```python
from build123d import *

# Parameters (mm, degrees)
F0_W      = 70
F0_H      = 70
F1_DEPTH  = 120
F3_D      = 13.49248
F4_D      = 8.8
F4_DEPTH  = 20
F4_TIP    = 2.6437867237
F2_R      = 15.05
F5_DEPTH  = 1.2
F7_D      = 8.8
F7_DEPTH  = 20
F7_TIP    = 2.6437867237
F6_R      = 15.05
F8_DEPTH  = 1.2
F10_D     = 5.5
F10_DEPTH = 20
F10_TIP   = 1.6523667023
F12_D     = 8.8
F12_DEPTH = 20
F12_TIP   = 2.6437867237
F14_D     = 10.0838
F14_DEPTH = 40
F14_TIP   = 3.0294791551
F13_R     = 13.75
F15_DEPTH = 1.2
F16_R     = 15.5
F17_DEPTH = 2


with BuildPart() as f1:
    # F0 (on Right) → F1 (new body)
    with BuildSketch(Plane.YZ):
        Rectangle(F0_W, F0_H)
    extrude(amount=F1_DEPTH)

    # F3 (through all)
    with Locations(Plane.YZ.offset(120)):
        with Locations((-19, 0), (19, 0)):
            Hole(F3_D / 2)

    # F4
    with Locations(Plane.YZ.offset(120)):
        with Locations((-26, 26), (26, 25.9378720075), (-18, -26), (18, -26)):
            Hole(F4_D / 2, depth=F4_DEPTH)
            with Locations((0, 0, -(F4_DEPTH + F4_TIP / 2))):  # 118° drill point
                Cone(0, F4_D / 2, F4_TIP, mode=Mode.SUBTRACT)

    # F2 (on face) → F5 (cut)
    with BuildSketch(Plane.YZ.offset(120)):
        with Locations((-19, 0)):
            Circle(F2_R)
        with Locations((19, 0)):
            Circle(F2_R)
    extrude(amount=-F5_DEPTH, mode=Mode.SUBTRACT)

    # F7
    with Locations(Plane(origin=(0, 0, 0), x_dir=(0, -1, 0), z_dir=(-1, 0, 0))):
        with Locations((-26, 25.9378720075), (26, 26), (-18, -26), (18, -26)):
            Hole(F7_D / 2, depth=F7_DEPTH)
            with Locations((0, 0, -(F7_DEPTH + F7_TIP / 2))):  # 118° drill point
                Cone(0, F7_D / 2, F7_TIP, mode=Mode.SUBTRACT)

    # F6 (on face) → F8 (cut)
    with BuildSketch(Plane(origin=(0, 0, 0), x_dir=(0, -1, 0), z_dir=(-1, 0, 0))):
        with Locations((-19, 0)):
            Circle(F6_R)
        with Locations((19, 0)):
            Circle(F6_R)
    extrude(amount=-F8_DEPTH, mode=Mode.SUBTRACT)

    # F10
    with Locations(Plane.XY.offset(35)):
        with Locations((19.5, 20.25), (19.5, -20.25), (50.5, -20.25), (50.5, 20.25), (69.5, 20.25), (69.5, -20.25), (100.5, -20.25), (100.5, 20.25)):
            Hole(F10_D / 2, depth=F10_DEPTH)
            with Locations((0, 0, -(F10_DEPTH + F10_TIP / 2))):  # 118° drill point
                Cone(0, F10_D / 2, F10_TIP, mode=Mode.SUBTRACT)

    # F12
    with Locations(Plane(origin=(0, 0, -35), x_dir=(1, 0, 0), z_dir=(0, 0, -1))):
        with Locations((8, 27), (8, -27), (112, 27), (112, -27)):
            Hole(F12_D / 2, depth=F12_DEPTH)
            with Locations((0, 0, -(F12_DEPTH + F12_TIP / 2))):  # 118° drill point
                Cone(0, F12_D / 2, F12_TIP, mode=Mode.SUBTRACT)

    # F14
    with Locations(Plane(origin=(0, 35, 0), x_dir=(-1, 0, 0), z_dir=(0, 1, 0))):
        with Locations((-85, 19), (-35, 19), (-35, -19), (-85, -19)):
            Hole(F14_D / 2, depth=F14_DEPTH)
            with Locations((0, 0, -(F14_DEPTH + F14_TIP / 2))):  # 118° drill point
                Cone(0, F14_D / 2, F14_TIP, mode=Mode.SUBTRACT)

    # F13 (on face) → F15 (cut)
    with BuildSketch(Plane(origin=(0, 35, 0), x_dir=(-1, 0, 0), z_dir=(0, 1, 0))):
        with Locations((-85, 19)):
            Circle(F13_R)
        with Locations((-85, -19)):
            Circle(F13_R)
        with Locations((-35, 19)):
            Circle(F13_R)
        with Locations((-35, -19)):
            Circle(F13_R)
    extrude(amount=-F15_DEPTH, mode=Mode.SUBTRACT)

    # F16 (on face) → F17 (cut)
    with BuildSketch(Plane.XZ.offset(35)):
        with Locations((67.5, -19)):
            Circle(F16_R)
    extrude(amount=-F17_DEPTH, mode=Mode.SUBTRACT)


solid = f1.part
```
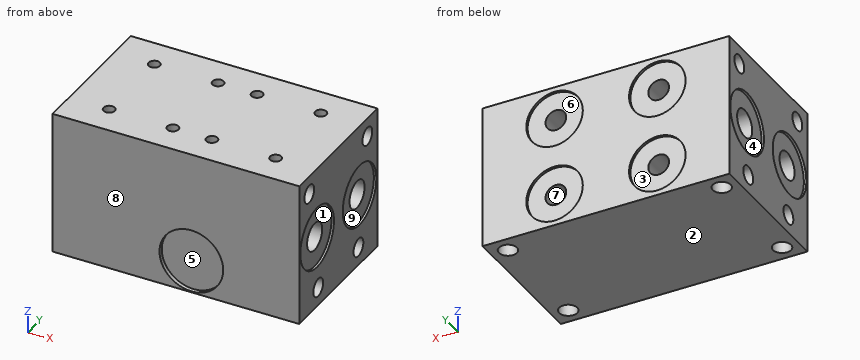
Verification items for the finished model (mm, model axes). Face numbers are marked on the shaded views. A direction names the side the tool comes from. Give positions to 0.01 mm unless a question says otherwise; leave off trailing zeros. Order: outer loops, then holes, each group sorted by start corner. A loop starts at its lowest first (then second) coordinate and runs counter-clockwise, first axis right, second up. Notation, with made-up numbers: (47, -23.75) -> (82, -23.75) arc R17 ccw to (82, -14.75) -> close; hole circle Ø6 at (68.25, 6). An arc over 180 degrees is marked (long way). One line per item, written item: value.
(1) Scan lines: line 1 along X through (y, z) = (-20, 28); line 2 along Y through (x, z) = (14, 29); line 3 along Y through (x, z) = (21, -27.5). Record each from-to range of solid material in increasing order. Write a range as [from, to].
Final values:
line 1: [0, 16.76], [22.24, 47.76], [53.24, 66.76], [72.24, 97.76], [103.24, 120]
line 2: [-35, -29.22], [-22.78, 22.84], [29.16, 35]
line 3: [-35, -20.29], [-15.71, 15.71], [20.29, 35]
(2) Sectioned sample at B-B on x = 24. Record the cut outline in (y, z), then the cut area to 3 significant figures.
Final values:
outline: (-35, -35) -> (35, -35) -> (35, -27.25) -> (33.8, -27.25) -> (33.8, -10.75) -> (35, -10.75) -> (35, 10.75) -> (33.8, 10.75) -> (33.8, 27.25) -> (35, 27.25) -> (35, 35) -> (-35, 35) -> close; hole circle Ø13.49 at (-19, 0); hole circle Ø13.49 at (19, 0)
area: 4,570 mm^2
(3) Sectioned sample at C-C on y = 28.5. Count the separate pieces of the cut face and the enclosed holes in it, then the cut area to 3 significant figures.
Final values:
separate pieces: 1
enclosed holes: 4
area: 7,380 mm^2
(4) Sectioned sample at A-A on z = 0. Record the cut outline in (x, y), then the cut area to 3 significant figures.
Final values:
outline: (0, -35) -> (120, -35) -> (120, -34.05) -> (118.8, -34.05) -> (118.8, -25.75) -> (1.2, -25.75) -> (1.2, -34.05) -> (0, -34.05) -> close; (0, -3.95) -> (1.2, -3.95) -> (1.2, -12.25) -> (118.8, -12.25) -> (118.8, -3.95) -> (120, -3.95) -> (120, 3.95) -> (118.8, 3.95) -> (118.8, 12.25) -> (1.2, 12.25) -> (1.2, 3.95) -> (0, 3.95) -> close; (0, 34.05) -> (1.2, 34.05) -> (1.2, 25.75) -> (118.8, 25.75) -> (118.8, 34.05) -> (120, 34.05) -> (120, 35) -> (0, 35) -> close
area: 5,080 mm^2
(5) Gauge pin test, flat ends, axial feed: pin 1 (7 mm diameter, centred on y = -26, z = 26, fed in from -X); pin 2 (24 mm diameter, centred on y = 19, z = 0, fed in from -X); pin 3 (22 mm diameter, centred on x = 35, z = -19, fed in from +Y). Record the tip position at first contact, or that the pin passes through.
Final values:
pin 1: x = 20.54
pin 2: x = 1.2
pin 3: y = 33.8
(6) Sectioned sample at D-D on x = 41.5. Record the cut outline in (y, z), then the cut area to 3 significant figures.
Final values:
outline: (-35, -35) -> (35, -35) -> (35, -31.12) -> (33.8, -31.12) -> (33.8, -6.88) -> (35, -6.88) -> (35, 6.88) -> (33.8, 6.88) -> (33.8, 31.12) -> (35, 31.12) -> (35, 35) -> (-35, 35) -> close; hole circle Ø13.49 at (-19, 0); hole circle Ø13.49 at (19, 0)
area: 4,560 mm^2
(7) Tool access check on the marked faces 1, 2, 3, 4 and 5. Record the directions out of +Z, -Z, +X, -X, +Y, -Y that give a thin tool (end or side, any length) a straight path to the whole face; none if there is none.
Final values:
face 1: +X
face 2: -Z, +X, -X, +Y, -Y
face 3: +Y
face 4: -X
face 5: -Y
(8) Draft check along Y on the marked faces 6, 7, 8 and 9. Enter one of: pulls with the +Y half, pulls with the -Y half, needs draft (parallel to the pull), parting line crosses it, or undercut.
Final values:
face 6: pulls with the +Y half
face 7: needs draft
face 8: pulls with the -Y half
face 9: undercut
